Model file for the job. Use its own axes, mm. A direction names the side the tool comes from. Coordinates: 2 decimals unless noted, no trailing zeros. Order: outer loops, then holes, each group sorted by start corner. A loop starts at its lowest first (then second) coordinate and runs counter-clockwise, first axis right, second up. Notation, with made-up numbers: (2.5, 68) - (45.5, 68) arc R32 cw to (45.5, 98) - close; hole circle Ø8 at (41, -18). An arc over 180 degrees is marked (long way). Put each result on its own line as item: value. Start each with the question number.
```python
from build123d import *

# Parameters (mm, degrees)
CROQUIS1_R              = 2.5
SALIENTE_EXTRUIR1_DEPTH = 10
CROQUIS2_R              = 1.5
CORTAR_EXTRUIR1_DEPTH   = 0.9
REDONDEO1_R             = 0.1
CROQUIS3_W              = 11
CROQUIS3_H              = 10
SALIENTE_EXTRUIR2_DEPTH = 10
CORTAR_EXTRUIR2_DEPTH   = 24.430749028
SALIENTE_EXTRUIR3_DEPTH = 10


with BuildPart() as part:
    # Croquis1 → Saliente-Extruir1 (new body)
    with BuildSketch(Plane.XY):
        Circle(CROQUIS1_R)
    extrude(amount=SALIENTE_EXTRUIR1_DEPTH)

    # Croquis2 → Cortar-Extruir1 (cut)
    with BuildSketch(Plane(origin=(0, 0, 0), x_dir=(-1, 0, 0), z_dir=(0, 0, -1))):
        Circle(CROQUIS2_R)
    extrude(amount=-CORTAR_EXTRUIR1_DEPTH, mode=Mode.SUBTRACT)

    # Redondeo1
    redondeo1_edges = [part.edges().sort_by_distance(p)[0] for p in [
        (1.5, 0, 0.9),
    ]]
    fillet(redondeo1_edges, radius=REDONDEO1_R)

    # Croquis3 → Saliente-Extruir2 (add)
    with BuildSketch(Plane.XY.offset(10)):
        with Locations((1.5, 0)):
            Rectangle(CROQUIS3_W, CROQUIS3_H)
    extrude(amount=SALIENTE_EXTRUIR2_DEPTH)

    # Croquis4 → Cortar-Extruir2 (cut, through all)
    with BuildSketch(Plane.XZ.offset(5)):
        with BuildLine():
            Line((-4, 20), (-4, 10))
            ThreePointArc((-4, 10), (1.453300741, 14.331864296), (5.5, 20))
            Line((5.5, 20), (-4, 20))
        make_face()
    extrude(amount=-CORTAR_EXTRUIR2_DEPTH, mode=Mode.SUBTRACT)

    # Croquis5 → Saliente-Extruir3 (add)
    with BuildSketch(Plane(origin=(0, 0, 0), x_dir=(-1, 0, 0), z_dir=(0, 0, -1))):
        with BuildLine():
            Line((0, -2.5), (-7, -2.5))
            Line((-7, -2.5), (-7, 2.5))
            Line((-7, 2.5), (0, 2.5))
            ThreePointArc((0, 2.5), (-2.5, 0), (0, -2.5))
        make_face()
    extrude(amount=-SALIENTE_EXTRUIR3_DEPTH)


solid = part.part
```
Item 1: Slice it at C-C, the plane z = 8.25. Give the cut face in (x, y).
Item 2: Flat gauge pins, fed straight in: pin 1 Ø3 at (x, y) = (3, 0) entering from +Z; pin 2 Ø5 at (x, y) = (6, 2.5) entering from -Z; pin 3 Ø6 at (x, z) = (1, 2.5) entering from +Y; pin 4 Ø3 at (x, z) = (2, 3.5) entering from -Y. Where does each tip first touch, or does it go through?
Item 3: 3-axis set-ups, long thin cutter, end or side, ignore diameter. For faces 1 (the face through (0, 0, 0.9)), 2 (the face through (4, 5, 14)), 3 (the face through (0, 3, 10)), 4 (the face through (3, -2.5, 5)): which of +Z, -Z, +X, -X, +Y, -Y reach the whole face in a straight line?
Item 4: Pull direction Y, two halves, no side cores. Call faces 5 (the face through (1.5, 0.07, 0.39)), 6 (the face through (4, 2.5, 5)), 7 (the face through (6, 0, 20)): pulls with the +Y half, pulls with the -Y half, needs draft (parallel to the pull), parting line crosses it, or undercut.
Item 5: Wall check: line 1 along Y through (x, z) = (-2, 6); line 2 along Y through (x, z) = (4.25, 6.75); line 3 along Z through (x, y) = (0.5, 3). Give the ranges that are in metal, low to high.
Item 6: Slice it at A-A, the plane y = 0. Give the cut face in (x, z), plus the area to 3 significant figures.
Item 7: Slice it at B-B, the plane x = 2.5. Give the cut face in (y, z), plus the area to 3 significant figures.
Item 8: Slice it at D-D, the plane y = 1.75. Give the cut face in (x, z), plus the area to 3 significant figures.
Here are the results:
1. outline: (0, -2.5) - (7, -2.5) - (7, 2.5) - (0, 2.5) arc R2.5 ccw to start
2. pin 1: stops at z = 18.26
2. pin 2: stops at z = 0
2. pin 3: stops at y = 2.5
2. pin 4: stops at y = -2.5
3. face 1: -Z
3. face 2: +Z, -Z, +X, -X, +Y
3. face 3: -Z, -X
3. face 4: -Z, +X, -X, -Y
4. face 5: undercut
4. face 6: pulls with the +Y half
4. face 7: needs draft
5. line 1: y = -1.5 to 1.5
5. line 2: y = -2.5 to 2.5
5. line 3: z = 10 to 13.38
6. outline: (-4, 10) - (-2.5, 10) - (-2.5, 0) - (-1.5, 0) - (-1.5, 0.8) arc R0.1 cw to (-1.4, 0.9) - (1.4, 0.9) arc R0.1 cw to (1.5, 0.8) - (1.5, 0) - (7, 0) - (7, 20) - (5.5, 20) arc R25 cw to start
6. area: 146 mm^2
7. outline: (-5, 10) - (-2.5, 10) - (-2.5, 0) - (2.5, 0) - (2.5, 10) - (5, 10) - (5, 15.51) - (-5, 15.51) - close
7. area: 105 mm^2
8. outline: (-4, 10) - (-1.79, 10) - (-1.79, 0) - (7, 0) - (7, 20) - (5.5, 20) arc R25 cw to start
8. area: 141 mm^2
